from build123d import *

# Parameters (mm, degrees)
SKETCH1_R           = 4
BOSS_EXTRUDE1_DEPTH = 325
CUT_EXTRUDE1_DEPTH  = 7.5
SKETCH3_R           = 4
SKETCH3_R_2         = 3.5
CUT_EXTRUDE2_DEPTH  = 1
SKETCH5_R           = 4
CUT_EXTRUDE3_DEPTH  = 65
SKETCH6_R           = 4
BOSS_EXTRUDE2_DEPTH = 13
SKETCH7_R           = 4
BOSS_EXTRUDE3_DEPTH = 10
SKETCH8_R           = 4
BOSS_EXTRUDE4_DEPTH = 40
SKETCH9_R           = 4
CUT_EXTRUDE4_DEPTH  = 30


with BuildPart() as part:
    # Sketch1 → Boss-Extrude1 (new body)
    with BuildSketch(Plane.XY):
        Circle(SKETCH1_R)
    extrude(amount=BOSS_EXTRUDE1_DEPTH)

    # Sketch2 → Cut-Extrude1 (cut)
    with BuildSketch(Plane.XY.offset(325)):
        with BuildLine():
            Line((3.122498999, 2.5), (-3.122498999, 2.5))
            ThreePointArc((-3.122498999, 2.5), (0, 4), (3.122498999, 2.5))
        make_face()
    extrude(amount=-CUT_EXTRUDE1_DEPTH, mode=Mode.SUBTRACT)

    # Sketch3 → Cut-Extrude2 (cut)
    with BuildSketch(Plane.XY.offset(323.75)):
        Circle(SKETCH3_R)
        Circle(SKETCH3_R_2, mode=Mode.SUBTRACT)
    extrude(amount=-CUT_EXTRUDE2_DEPTH, mode=Mode.SUBTRACT)

    # Sketch5 → Cut-Extrude3 (cut)
    with BuildSketch(Plane(origin=(0, 0, 0), x_dir=(-1, 0, 0), z_dir=(0, 0, -1))):
        Circle(SKETCH5_R)
    extrude(amount=-CUT_EXTRUDE3_DEPTH, mode=Mode.SUBTRACT)

    # Sketch6 → Boss-Extrude2 (add)
    with BuildSketch(Plane(origin=(0, 0, 65), x_dir=(-1, 0, 0), z_dir=(0, 0, -1))):
        Circle(SKETCH6_R)
    extrude(amount=BOSS_EXTRUDE2_DEPTH)

    # Sketch7 → Boss-Extrude3 (add)
    with BuildSketch(Plane(origin=(0, 0, 52), x_dir=(-1, 0, 0), z_dir=(0, 0, -1))):
        Circle(SKETCH7_R)
    extrude(amount=BOSS_EXTRUDE3_DEPTH)

    # Sketch8 → Boss-Extrude4 (add)
    with BuildSketch(Plane(origin=(0, 0, 42), x_dir=(-1, 0, 0), z_dir=(0, 0, -1))):
        Circle(SKETCH8_R)
    extrude(amount=BOSS_EXTRUDE4_DEPTH)

    # Sketch9 → Cut-Extrude4 (cut)
    with BuildSketch(Plane(origin=(0, 0, 2), x_dir=(-1, 0, 0), z_dir=(0, 0, -1))):
        Circle(SKETCH9_R)
    extrude(amount=-CUT_EXTRUDE4_DEPTH, mode=Mode.SUBTRACT)


solid = part.part
Geometry: final body of the model. Coordinates: model frame, mm. A direction names the side the tool comes from. Round coordinates to 2 decimals unless told otherwise and drop trailing zeros. Loops run counter-clockwise (first coordinate to the right, second up) from the corner with the lowest first, then second, coordinate; pieces in that order, holes last.
Q1. Section A-A on z = 152. Return loops of the section in (x, y), plus the area to 3 significant figures.
Q2. Material intervals for L1, parallel to Z at x = 3.5, y = 1.25; L2, parallel to Y at x = -0.25, z = 211; L3, parallel to Y at x = 2.5, z = 174, sorted ascending.
Q3. Access query for faces 1 (the flat face through (0, -1, 325)), 2 (the flat face through (0, 2.5, 321)). Directions: +Z, -Z, +X, -X, +Y, -Y. A direction counts if a zero-diameter tool reaches every point of the face in a straight line with its end or side. Return the directions, or none.
Q4. Pin query (flat end, axial travel): P1, Ø1.5, axis at x = -2, z = 135.5, coming from the -Y side; P2, Ø0.8, axis at x = 0, y = 3.5, coming from the +Z side. Return the tip coordinate at first contact, or that it passes through.
Q5. Pull-direction query (Z, two-part tool) for faces 3 (the cylindrical face through (-0.1, -3.5, 323.3)), 4 (the cylindrical face through (0, -4, 324)), 5 (the flat face through (-0.61, -3.62, 323.75)), 6 (the flat face through (0, 0, 32)); classes: released by +Z, released by -Z, zero draft, split by the parting line, or undercut.
Evaluation:
1. outline: circle Ø8 at (0, 0)
1. area: 50.3 mm2
2. L1: z = 32 to 322.75, 323.75 to 325
2. L2: y = -3.99 to 3.99
2. L3: y = -3.12 to 3.12
3. face 1: +Z, +X, -X, +Y, -Y
3. face 2: +Z, +X, -X, +Y
4. P1: stops at y = -3.8
4. P2: stops at z = 317.5
5. face 3: undercut
5. face 4: zero draft
5. face 5: undercut
5. face 6: released by -Z
